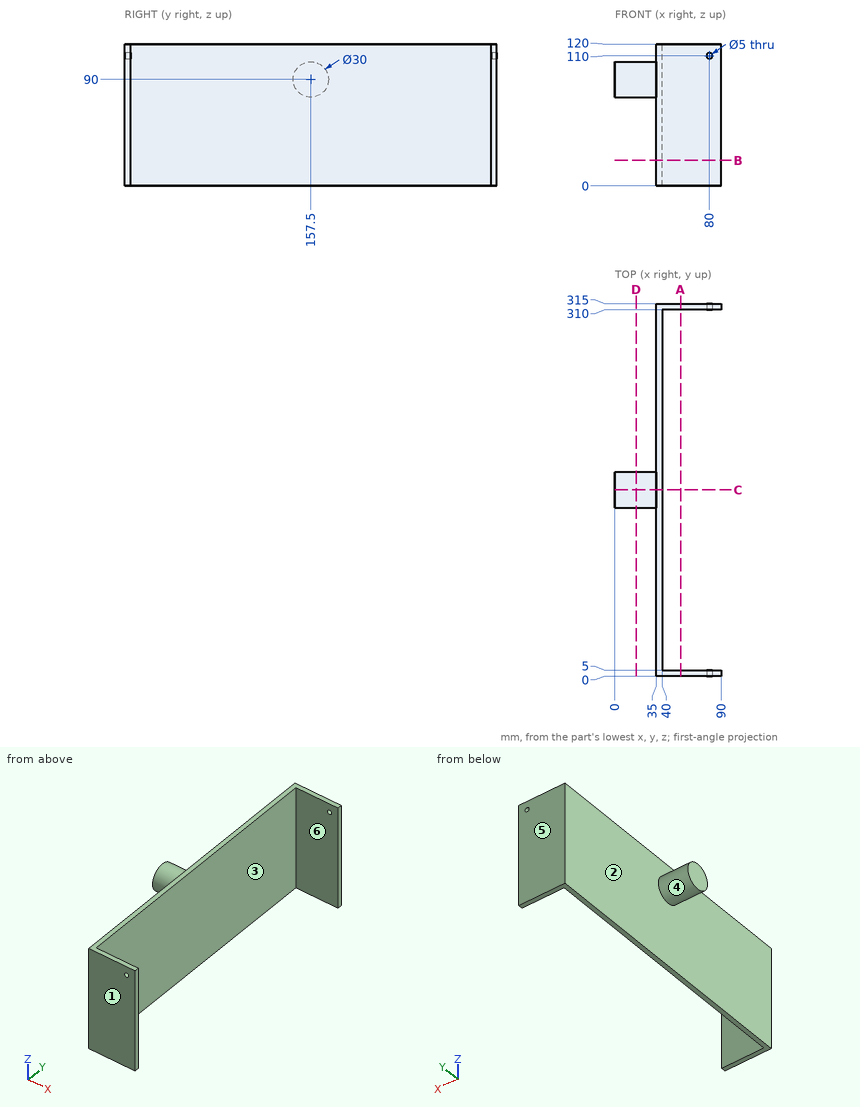
Source: three-view drawing plus pictorial views. Frame: mm from the lowest corner of the part. A direction names the side the tool comes from. Coordinates: 2 decimals unless noted, no trailing zeros. Order: outer loops, then holes, each group sorted by start corner. A loop starts at its lowest first (then second) coordinate and runs counter-clockwise, first axis right, second up.
1) Ray query, probe 1 along X at (y, z) = (311.65, 110); probe 2 along Y at (x, z) = (60, 91); probe 3 along Z at (x, y) = (80, 4). Return the intervals inside material, ascending.
Result sheet:
probe 1: x = 35 to 77.5, 82.5 to 90
probe 2: y = 0 to 5, 310 to 315
probe 3: z = 0 to 107.5, 112.5 to 120
2) First-contact query: P1, Ø1, axis at x = 20, z = 79.5, coming from the +Y side; P2, Ø10, axis at y = 121, z = 72.5, coming from the +X side; P3, Ø5, axis at y = 59.5, z = 65, coming from the -X side. Flat tips, straight axial feed; report the tip coordinate or a pass-through.
Result sheet:
P1: stops at y = 168.68
P2: stops at x = 40
P3: stops at x = 35
3) Section D-D (x = 18). Return loops of the section in (y, z).
Result sheet:
outline: circle Ø30 at (157.5, 90)
4) Section C-C (y = 157.5). Return loops of the section in (x, z), then the cut area to 3 significant figures.
Result sheet:
outline: (0, 75) - (35, 75) - (35, 0) - (40, 0) - (40, 120) - (35, 120) - (35, 105) - (0, 105) - close
area: 1,650 mm2
5) Set-up query: the marked faces 4, 5 and 6. Return all of +Z, -Z, +X, -X, +Y, -Y with unobstructed straight access to the full face (end or side cutting, diameter ignored); none if empty.
Result sheet:
face 4: -X
face 5: +Z, -Z, +X, -X, +Y
face 6: +Z, -Z, +X
6) Section B-B (z = 21.5). Return loops of the section in (x, y).
Result sheet:
outline: (35, 0) - (90, 0) - (90, 5) - (40, 5) - (40, 310) - (90, 310) - (90, 315) - (35, 315) - close
7) Draft query along Y for the marked faces 1, 2 and 3. Return one class per face: released by +Y, released by -Y, zero draft, split by the parting line, or undercut.
Result sheet:
face 1: released by -Y
face 2: zero draft
face 3: undercut
8) Section A-A (x = 55.5). Return loops of the section in (y, z).
Result sheet:
outline: (0, 0) - (5, 0) - (5, 120) - (0, 120) - close; (310, 0) - (315, 0) - (315, 120) - (310, 120) - close
